Design review of the part built by this model. Coordinates are the model's own, in mm. A direction names the side the tool comes from. Coordinates: 2 decimals unless noted, no trailing zeros. Write each loop counter-clockwise with the first axis right and the second up, starting at its lowest first coordinate (ties: lowest second). Pieces come first, ordered by that corner, then holes.
Q1. Machinability: for faces 1 (the face through (0.21, 249.75, -6.49)), 2 (the face through (0, -3, 5.5)), which of the approach directions +Z, -Z, +X, -X, +Y, -Y give a long, thin tool a straight path to every point of the face, cutting with its end or side? Answer none if there is none.
Q2. Add section A-A, the plane y = -168.5. Give the boundary of the cut face in (x, z), plus the area to 3 significant figures.
Q3. To check wall thickness, follow probe 1 along X at (y, z) = (-188, 2.25); probe 2 along Z at (x, y) = (-3, -56); probe 3 along Z at (x, y) = (-12.5, -218). State the ranges of each line that lie inside material, in increasing order.
Q4. Add section B-B, the plane x = -1.5. Give the boundary of the cut face in (y, z), plus the area to 3 significant figures.
Q5. The part is to be moulded in two halves that separate along Z. For faces 3 (the face through (0.21, -249.75, -6.49)), 4 (the face through (0, -4, -7.5)), 5 (the face through (0, -3, -5.5)), say which applies: +Z half, -Z half, draft (parallel to the pull), parting line (faces both ways), or undercut.
Q6. Clearance check with flat-ended pins moving along their axes: pin 1 Ø5 at (x, z) = (-4.5, -4.5) entering from +Y; pin 2 Ø5 at (x, z) = (2, -6) entering from +Y; pin 3 Ø1 at (y, z) = (-179, -5) entering from -X. State where each tip first meets the part, or that it passes through.
Q7. Add section C-C, the plane z = 0.5. Give the boundary of the cut face in (x, y), plus the area to 3 significant figures.
from build123d import *

# Parameters (mm, degrees)
EXTRUDE_1_DEPTH      = 250
EXTRUDE_1_DEPTH_BACK = 250
CHAMFER_1_SIZE       = 4
CHAMFER_1_SIZE_2     = 14.92820323


with BuildPart() as part:
    # Эскиз1 → Вытянуть-Тонкостенный1 (new, two sides: drawn at the far end of the back side and taken through both)
    with BuildSketch(Plane(origin=(0, 0, 0), x_dir=(1, 0, 0), z_dir=(0, 1, 0)).offset(-EXTRUDE_1_DEPTH_BACK)):
        with BuildLine():
            Line((-11, 7.5), (11, 7.5))
            ThreePointArc((11, 7.5), (13.828427125, 6.328427125), (15, 3.5))
            Line((15, 3.5), (15, -3.5))
            ThreePointArc((15, -3.5), (13.828427125, -6.328427125), (11, -7.5))
            Line((11, -7.5), (-11, -7.5))
            ThreePointArc((-11, -7.5), (-13.828427125, -6.328427125), (-15, -3.5))
            Line((-15, -3.5), (-15, 3.5))
            ThreePointArc((-15, 3.5), (-13.828427125, 6.328427125), (-11, 7.5))
        make_face()
        with BuildLine():
            Line((-11, 5.5), (11, 5.5))
            ThreePointArc((11, 5.5), (12.414213562, 4.914213562), (13, 3.5))
            Line((13, 3.5), (13, -3.5))
            ThreePointArc((13, -3.5), (12.414213562, -4.914213562), (11, -5.5))
            Line((11, -5.5), (-11, -5.5))
            ThreePointArc((-11, -5.5), (-12.414213562, -4.914213562), (-13, -3.5))
            Line((-13, -3.5), (-13, 3.5))
            ThreePointArc((-13, 3.5), (-12.414213562, 4.914213562), (-11, 5.5))
        make_face(mode=Mode.SUBTRACT)
    extrude(amount=EXTRUDE_1_DEPTH + EXTRUDE_1_DEPTH_BACK)

    # Фаска1
    # the kernel refuses this chamfer: 14.92820323, 4 mm, written as the material it takes off along each edge
    with BuildSketch(Plane(origin=(49.764387332, -250, 7.5), x_dir=(0, 0.9905000388259542, 0.13751244702129073), z_dir=(-1, 0, 0))) as chamfer_1_piece_1:
        Polygon((CHAMFER_1_SIZE * 0.990500038826, CHAMFER_1_SIZE * 0.137512447021), (-CHAMFER_1_SIZE_2 * 0.137512447024, CHAMFER_1_SIZE_2 * 0.990500038844), (0, 0), align=None)
    extrude(amount=99.528774665, mode=Mode.SUBTRACT)
    with BuildSketch(Plane(origin=(49.764387332, 250, 7.5), x_dir=(0, -0.9905000388259542, 0.13751244702129073), z_dir=(-1, 0, 0))) as chamfer_1_piece_2:
        Polygon((CHAMFER_1_SIZE * 0.990500038826, -CHAMFER_1_SIZE * 0.137512447021), (-CHAMFER_1_SIZE_2 * 0.137512447024, -CHAMFER_1_SIZE_2 * 0.990500038844), (0, 0), align=None)
    extrude(amount=99.528774665, mode=Mode.SUBTRACT)


solid = part.part
Here are the results:
1. face 1: +Z, +X, -X, +Y
1. face 2: +Y, -Y
2. outline: (-15, -3.5) arc R4 ccw to (-11, -7.5) - (11, -7.5) arc R4 ccw to (15, -3.5) - (15, 3.5) arc R4 ccw to (11, 7.5) - (-11, 7.5) arc R4 ccw to (-15, 3.5) - close; hole (-13, -3.5) arc R2 ccw to (-11, -5.5) - (11, -5.5) arc R2 ccw to (13, -3.5) - (13, 3.5) arc R2 ccw to (11, 5.5) - (-11, 5.5) arc R2 ccw to (-13, 3.5) - close
2. area: 154 mm2
3. probe 1: x = -15 to -13, 13 to 15
3. probe 2: z = -7.5 to -5.5, 5.5 to 7.5
3. probe 3: z = -7.21 to -4.82, 4.82 to 7.21
4. outline: (-250, -7.5) - (250, -7.5) - (250, -7.43) - (249.48, -5.5) - (-249.48, -5.5) - (-250, -7.43) - close; (-246.54, 5.5) - (246.54, 5.5) - (246, 7.5) - (-246, 7.5) - close
4. area: 1,980 mm2
5. face 3: +Z half
5. face 4: -Z half
5. face 5: undercut
6. pin 1: stops at y = 249.89
6. pin 2: stops at y = 250
6. pin 3: stops at x = -14.87
7. outline: (-15, -247.88) - (-13, -247.88) - (-13, 247.88) - (-15, 247.88) - close; (13, -247.88) - (15, -247.88) - (15, 247.88) - (13, 247.88) - close
7. area: 1,980 mm2
